from build123d import *

# Parameters (mm, degrees)
RESSALTO_EXTRUS_O1_DEPTH    = 4
ESBO_O33_W                  = 8
ESBO_O33_H                  = 24.32835801
CORTE_EXTRUS_O20_DEPTH      = 59.436005136
CORTE_EXTRUS_O22_DEPTH      = 51.515563889
RESSALTO_EXTRUS_O14_DEPTH   = 4
ESBO_O38_R                  = 7
CORTE_EXTRUS_O23_DEPTH      = 39.915014679
ESBO_O39_W                  = 29.519685428
ESBO_O39_H                  = 8
CORTE_EXTRUS_O24_DEPTH      = 38.873187976
CORTE_EXTRUS_O25_DEPTH      = 39.915014679
CORTE_EXTRUS_O25_DEPTH_BACK = 39.915014679
ESBO_O40_W                  = 11.533486782
ESBO_O40_H                  = 2
CORTE_EXTRUS_O26_DEPTH      = 0.156854249
RESSALTO_EXTRUS_O15_START   = -1
RESSALTO_EXTRUS_O15_DEPTH   = 2
RESSALTO_EXTRUS_O16_START   = 2
RESSALTO_EXTRUS_O16_DEPTH   = 2
CORTE_EXTRUS_O27_DEPTH      = 43.203568046
CORTE_EXTRUS_O27_DEPTH_BACK = 43.203568046
ESBO_O44_R                  = 1.5


with BuildPart() as part:
    # Esboço1 → Ressalto-extrusão1 (new body)
    with BuildSketch(Plane.XY):
        with BuildLine():
            Line((40.514368641, 0), (48.514368641, 0))
            ThreePointArc((48.514368641, 0), (39.227067694, 12.823953684), (24.146045917, 8))
            Line((24.146045917, 8), (-21.519685428, 8))
            Line((-21.519685428, 8), (-21.519685428, 32.32835801))
            Line((-21.519685428, 32.32835801), (-29.519685428, 32.32835801))
            Line((-29.519685428, 32.32835801), (-29.519685428, 0))
            Line((-29.519685428, 0), (29.519685428, 0))
            ThreePointArc((29.519685428, 0), (35.017027034, 5.497341607), (40.514368641, 0))
        make_face()
    extrude(amount=RESSALTO_EXTRUS_O1_DEPTH)

    # Esboço33 → Corte-extrusão20 (cut, through all)
    with BuildSketch(Plane.XY.offset(4)):
        with Locations((-25.519685428, 20.164179005)):
            Rectangle(ESBO_O33_W, ESBO_O33_H)
    extrude(amount=-CORTE_EXTRUS_O20_DEPTH, mode=Mode.SUBTRACT)

    # Esboço34 → Corte-extrusão22 (cut, through all)
    with BuildSketch(Plane.XY.offset(4)):
        with BuildLine():
            Line((21.519685428, 0), (21.519685428, 8))
            Line((21.519685428, 8), (24.146045917, 8))
            ThreePointArc((24.146045917, 8), (39.227067694, 12.823953684), (48.514368641, 0))
            Line((48.514368641, 0), (40.514368641, 0))
            ThreePointArc((40.514368641, 0), (35.017027034, 5.497341607), (29.519685428, 0))
            Line((29.519685428, 0), (21.519685428, 0))
        make_face()
    extrude(amount=-CORTE_EXTRUS_O22_DEPTH, mode=Mode.SUBTRACT)

    # Esboço36 → Revolução1 (revolve)
    with BuildSketch(Plane.XY.offset(4)):
        with BuildLine():
            Line((27.019685428, -2), (27.019685428, -4))
            ThreePointArc((27.019685428, -4), (19.019685428, 4), (27.019685428, 12))
            Line((27.019685428, 12), (27.019685428, 10))
            ThreePointArc((27.019685428, 10), (21.019685428, 4), (27.019685428, -2))
        make_face()
    revolve(axis=Axis((27.019685428, -2, 4), (0, 1, 0)))

    # Esboço37 → Ressalto-extrusão14 (add)
    with BuildSketch(Plane.XY.offset(4)):
        with BuildLine():
            ThreePointArc((21.362831178, 8), (20.091482197, 4), (21.362831178, 0))
            Line((21.362831178, 0), (21.362831178, 8))
        make_face()
        with BuildLine():
            Line((20.091482197, 0), (21.362831178, 0))
            ThreePointArc((21.362831178, 0), (20.091482197, 4), (21.362831178, 8))
            Line((21.362831178, 8), (20.091482197, 8))
            Line((20.091482197, 8), (-29.519685428, 8))
            Line((-29.519685428, 8), (-29.519685428, 0))
            Line((-29.519685428, 0), (20.091482197, 0))
        make_face()
    extrude(amount=RESSALTO_EXTRUS_O14_DEPTH)

    # Esboço38 → Corte-extrusão23 (cut, through all)
    with BuildSketch(Plane(origin=(0, 0, 0), x_dir=(-1, 0, 0), z_dir=(0, 0, -1))):
        with Locations((-27.019685428, 4)):
            Circle(ESBO_O38_R)
    extrude(amount=CORTE_EXTRUS_O23_DEPTH, mode=Mode.SUBTRACT)

    # Esboço39 → Corte-extrusão24 (cut, through all)
    with BuildSketch(Plane.XY.offset(8)):
        with Locations((-14.759842714, 4)):
            Rectangle(ESBO_O39_W, ESBO_O39_H)
    extrude(amount=-CORTE_EXTRUS_O24_DEPTH, mode=Mode.SUBTRACT)

    # Esboço40 → Corte-extrusão25 (cut, two sides: drawn at the far end of the back side and taken through both)
    with BuildSketch(Plane(origin=(0, 0, 0), x_dir=(-1, 0, 0), z_dir=(0, 0, -1)).offset(-CORTE_EXTRUS_O25_DEPTH_BACK)):
        with Locations((-29.252942037, 4)):
            Rectangle(ESBO_O40_W, ESBO_O40_H)
    extrude(amount=CORTE_EXTRUS_O25_DEPTH + CORTE_EXTRUS_O25_DEPTH_BACK, mode=Mode.SUBTRACT)

    # Esboço41 → Corte-extrusão26 (cut)
    with BuildSketch(Plane(origin=(21.519685428, 0, 0), x_dir=(0, 0, -1), z_dir=(1, 0, 0))):
        with BuildLine():
            Line((-4, 6.397915762), (-4, 1.602084238))
            ThreePointArc((-4, 1.602084238), (-1.602084238, 4), (-4, 6.397915762))
        make_face()
    extrude(amount=-CORTE_EXTRUS_O26_DEPTH, mode=Mode.SUBTRACT)

    # Esboço42 → Ressalto-extrusão15 (add)
    with BuildSketch(Plane(origin=(0, 8, 0), x_dir=(1, 0, 0), z_dir=(0, 1, 0)).offset(RESSALTO_EXTRUS_O15_START)):
        with BuildLine():
            Line((32.597781304, 0), (38.266819794, 0))
            ThreePointArc((38.266819794, 0), (38.956939361, -4), (38.266819794, -8))
            Line((38.266819794, -8), (32.597781304, -8))
            ThreePointArc((32.597781304, -8), (33.88373333, -4), (32.597781304, 0))
        make_face()
    extrude(amount=-RESSALTO_EXTRUS_O15_DEPTH)

    # Esboço43 → Ressalto-extrusão16 (add)
    with BuildSketch(Plane.XZ.offset(-5).offset(RESSALTO_EXTRUS_O16_START)):
        with BuildLine():
            Line((38.266819794, 8), (33.264683426, 8))
            ThreePointArc((33.264683426, 8), (34.435883915, 4), (33.264683426, 0))
            Line((33.264683426, 0), (38.266819794, 0))
            ThreePointArc((38.266819794, 0), (38.956939361, 4), (38.266819794, 8))
        make_face()
    extrude(amount=RESSALTO_EXTRUS_O16_DEPTH)

    # Esboço44 → Corte-extrusão27 (cut, two sides: drawn at the far end of the back side and taken through both)
    with BuildSketch(Plane(origin=(0, 7, 0), x_dir=(1, 0, 0), z_dir=(0, 1, 0)).offset(-CORTE_EXTRUS_O27_DEPTH_BACK)):
        with Locations(Location((37.019685428, -4, 0), (0, 0, 90))):
            Circle(ESBO_O44_R)
    extrude(amount=CORTE_EXTRUS_O27_DEPTH + CORTE_EXTRUS_O27_DEPTH_BACK, mode=Mode.SUBTRACT)


solid = part.part
Model file for the job. Use its own axes, mm. A direction names the side the tool comes from. Round coordinates to 2 decimals unless told otherwise and drop trailing zeros. Loops run counter-clockwise (first coordinate to the right, second up) from the corner with the lowest first, then second, coordinate; pieces in that order, holes last.
1. Tool access for faces 1 (the cylindrical face through (38.957, 2.014, 3.943)), 2 (the flat face through (21.363, 4, 4)), 3 (the flat face through (33, 3, 6)): list every direction of +Z, -Z, +X, -X, +Y, -Y with a clear straight run to the whole face (end or side of a thin tool).
Check values:
face 1: +X, +Y, -Y
face 2: none
face 3: +Z, -Z, +X
2. Band-saw the part on D-D, the plane x = 3.5. List the corners of the cut face in (y, z), and give its area (3 significant figures).
Check values:
outline: (0, 0) - (8, 0) - (8, 8) - (0, 8) - close
area: 64.0 mm2
3. Drop flat-ended pins along their axis: P1, Ø1.7, axis at x = 35.5, z = 3, coming from the -Y side; P2, Ø5, axis at x = 37.02, z = 4, coming from the +Y side; P3, Ø2, axis at x = 37, y = 6, coming from the +Z side. Give the stop position or say it passes through.
Check values:
P1: stops at y = 1
P2: stops at y = 7
P3: stops at z = 8
4. Band-saw the part on C-C, the plane z = 1.25. List the corners of the cut face in (x, y), and give its area (3 significant figures).
Check values:
outline: (0, 0) - (20.66, 0) arc R7.51 ccw to (33.91, 1) - (38.64, 1) - (38.64, 3) - (32.26, 3) arc R5.33 cw (long way) to (32.26, 5) - (38.64, 5) - (38.64, 7) - (33.91, 7) arc R7.51 ccw to (20.66, 8) - (0, 8) - close
area: 260 mm2
5. Mould opens along X. For faces 4 (the cylindrical face through (35.532, 1.986, 4.195)), 5 (the cylindrical face through (38.957, 6.014, 3.943)), 6 (the flat face through (11, 0, 4)) say: +X half, -X half, draft (parallel to the pull), parting line (faces both ways), or undercut.
Check values:
face 4: undercut
face 5: +X half
face 6: draft
6. Wall check: probe 1 along Y at (x, z) = (34, 1); probe 2 along X at (y, z) = (5.8, 4); probe 3 along X at (y, z) = (2.5, 4). Give the ranges that are in metal, low to high.
Check values:
probe 1: y = 1 to 3, 5 to 7
probe 2: x = 0 to 21.36, 32.74 to 35.52, 38.52 to 38.96
probe 3: x = 0 to 21.36, 32.83 to 35.52, 38.52 to 38.96
7. Band-saw the part on B-B, the plane y = 4. List the corners of the cut face in (x, z).
Check values:
outline: (0, 0) - (22.55, 0) arc R6 cw to (21.52, 1.6) - (21.36, 1.6) - (21.36, 6) arc R6 cw to (23.49, 8.85) - (23.49, 11.18) arc R8 ccw to (20.09, 8) - (0, 8) - close
8. Band-saw the part on A-A, the plane x = 29. List the corners of the cut face in (y, z).
Check values:
outline: (-2.64, 0) - (-0.01, 0) arc R5.66 cw to (3, 9.57) - (3, 11.69) arc R7.75 ccw to start; (5, 9.57) arc R5.66 cw to (8.01, 0) - (10.64, 0) arc R7.75 ccw to (5, 11.69) - close
